```python
from build123d import *

# Parameters (mm, degrees)
F0_W        = 52.5702424347
F0_H        = 44.9169911444
F1_DEPTH    = 25
F2_DEPTH    = 25
F3_T        = -2.5
F4_SIZE     = 1
F5_T1_DEPTH = 68.9169911444
F5_T3_DEPTH = 6.1776694265
F5_T5_DEPTH = 48.0000001753
F5_T7_DEPTH = 6.1776694575
F5_T9_DEPTH = 75


# Not quite as in the source:
# - a fillet or chamfer that OpenCascade refuses, or shapes differently, is made with other operations: its cross-section is extruded or revolved along the edge and cut away or added


with BuildPart() as f1:
    # F0 (on Front) → F1 (new body)
    with BuildSketch(Plane.XZ):
        with Locations((26.2851212174, 22.4584955722)):
            Rectangle(F0_W, F0_H)
    extrude(amount=F1_DEPTH)

    # F2 (add): a face of the model
    f2_faces = [f1.faces().sort_by_distance(p)[0] for p in [
        (26.2851212174, -25, 22.4584955722),
    ]]
    extrude(f2_faces, amount=F2_DEPTH)

    # F3
    f3_openings = [f1.faces().sort_by_distance(p)[0] for p in [
        (26.285121, -25, 44.916991),
    ]]
    offset(amount=F3_T, openings=f3_openings)

    # F4
    f4_edges = [f1.edges().sort_by_distance(p)[0] for p in [
        (52.570242, 0, 22.458496),
        (52.570242, -25, 44.916991),
        (26.285121, -50, 44.916991),
        (0, -25, 44.916991),
        (26.285121, 0, 44.916991),
        (2.5, -25, 44.916991),
        (26.285121, -47.5, 44.916991),
        (50.070242, -25, 44.916991),
        (26.285121, -2.5, 44.916991),
    ]]
    chamfer(f4_edges, length=F4_SIZE)

    # F5: fillet of radius 5 on 4 edges, made by hand

    # F5_s2 → F5_t1 (cut)
    with BuildSketch(Plane.XY.offset(-12.5)):
        with BuildLine():
            ThreePointArc((0, -45), (1.4644660941, -48.5355339059), (5, -50))
            Line((5, -50), (0, -50))
            Line((0, -50), (0, -45))
        make_face()
        with BuildLine():
            ThreePointArc((0, -5), (1.4644660941, -1.4644660941), (5, 0))
            Line((5, 0), (0, 0))
            Line((0, 0), (0, -5))
        make_face()
    extrude(amount=F5_T1_DEPTH, mode=Mode.SUBTRACT)

    # F5_s4 → F5_t3 (cut)
    with BuildSketch(Plane.XZ.offset(49.0000001032)):
        with BuildLine():
            ThreePointArc((0, 41.8459233326), (0.3806023374, 43.7593404944), (1.4644660941, 45.3814572385))
            Line((1.4644660941, 45.3814572385), (0, 43.9169911444))
            Line((0, 43.9169911444), (0, 41.8459233326))
        make_face()
    extrude(amount=F5_T3_DEPTH, mode=Mode.SUBTRACT)

    # F5_s6 → F5_t5 (cut)
    with BuildSketch(Plane.XZ.offset(0.9999999279)):
        with BuildLine():
            ThreePointArc((0, 41.9169911444), (0.2565835097, 43.4981299745), (1, 44.9169911444))
            Line((1, 44.9169911444), (0, 43.9169911444))
            Line((0, 43.9169911444), (0, 41.9169911444))
        make_face()
    extrude(amount=F5_T5_DEPTH, mode=Mode.SUBTRACT)

    # F5_s8 → F5_t7 (cut)
    with BuildSketch(Plane.XZ.offset(-5.1776695297)):
        with BuildLine():
            ThreePointArc((0, 41.8459233326), (0.3806023374, 43.7593404944), (1.4644660941, 45.3814572385))
            Line((1.4644660941, 45.3814572385), (0, 43.9169911444))
            Line((0, 43.9169911444), (0, 41.8459233326))
        make_face()
    extrude(amount=F5_T7_DEPTH, mode=Mode.SUBTRACT)

    # F5_s10 → F5_t9 (cut)
    with BuildSketch(Plane.XZ.offset(-12.5)):
        with BuildLine():
            ThreePointArc((0, 5), (1.4644660941, 1.4644660941), (5, 0))
            Line((5, 0), (0, 0))
            Line((0, 0), (0, 5))
        make_face()
    extrude(amount=F5_T9_DEPTH, mode=Mode.SUBTRACT)


solid = f1.part
```
Read the model definition and answer for the solid it produces. Units are mm, in the model's axes. A direction names the side the tool comes from. Coordinates: 2 decimals unless noted, no trailing zeros. Write each loop counter-clockwise with the first axis right and the second up, starting at its lowest first coordinate (ties: lowest second). Pieces come first, ordered by that corner, then holes. Notation, with made-up numbers: (-32, 55) -> (-10, 55) arc R34 ccw to (-10, 85) -> close; hole circle Ø1 at (40, -0.5). An arc over 180 degrees is marked (long way). Answer as a JSON object with one key per item and string values.
Q1. The part is cut by section D-D on y = -4. Give the vertices of the cut face in (x, z).
The answers:
{"outline": "(0.1, 4) arc R5 ccw to (5, 0) -> (52.57, 0) -> (52.57, 43.92) -> (51.57, 44.92) -> (51.07, 44.92) -> (50.07, 43.92) -> (50.07, 2.5) -> (2.5, 2.5) -> (2.5, 43.92) -> (1.5, 44.92) -> (1, 44.92) arc R5 ccw to (0.1, 42.92) -> close"}
Q2. Consider line 1 (X direction, y = -42.5, z = 32); line 2 (Y direction, x = 16, z = 10.5); line 3 (Z direction, x = 6, y = -32). Determine where each line is inside the solid, lowest interval first. Write a range as [from, to].
The answers:
{"line 1": "x = [0, 2.5], [50.07, 52.57]", "line 2": "y = [-50, -47.5], [-2.5, 0]", "line 3": "z = [0, 2.5]"}
Q3. Flat-ended cylindrical pins translate along their axes: pin 1 Ø5 at (x, y) = (44, -8) entering from +Z; pin 2 Ø12 at (x, y) = (36.5, -26) entering from -Z. Find the tip coordinate at first contact, or state that the pin passes through.
The answers:
{"pin 1": "stops at z = 2.5", "pin 2": "stops at z = 0"}
Q4. Determine the mould class of faces 3 (the cylindrical face through (0.25, -24.68, 43.48)), 4 (the flat face through (28, -50, 22)), 5 (the flat face through (26, -25, 2.5)) for opening direction X: pulls with the +X half, pulls with the -X half, needs draft (parallel to the pull), parting line crosses it, or undercut.
The answers:
{"face 3": "pulls with the -X half", "face 4": "needs draft", "face 5": "undercut"}
Q5. A tool of negligible diameter and unlimited length cuts with its end or side. For faces 1 (the flat face through (26, -2.5, 23)), 2 (the flat face through (28, -25, 0)), from which of +Z, -Z, +X, -X, +Y, -Y can it reach the whole face along a straight path? Write none if from no direction.
The answers:
{"face 1": "+Z", "face 2": "-Z, +X, -X, +Y, -Y"}
Q6. The part is cut by section A-A on x = 8.5. Give the vertices of the cut face in (y, z).
The answers:
{"outline": "(-50, 0) -> (0, 0) -> (0, 43.92) -> (-1, 44.92) -> (-1.5, 44.92) -> (-2.5, 43.92) -> (-2.5, 2.5) -> (-47.5, 2.5) -> (-47.5, 43.92) -> (-48.5, 44.92) -> (-49, 44.92) -> (-50, 43.92) -> close"}
Q7. The part is cut by section C-C on y = -37. Give the vertices of the cut face in (x, z), then the cut area to 3 significant figures.
The answers:
{"outline": "(0, 5) arc R5 ccw to (5, 0) -> (52.57, 0) -> (52.57, 43.92) -> (51.57, 44.92) -> (51.07, 44.92) -> (50.07, 43.92) -> (50.07, 2.5) -> (2.5, 2.5) -> (2.5, 43.92) -> (1.5, 44.92) -> (1, 44.92) arc R5 ccw to (0, 41.92) -> close", "area": "336 mm2"}
Q8. The part is cut by section B-B on z = 37. Give the vertices of the cut face in (x, y), then the cut area to 3 significant figures.
The answers:
{"outline": "(0, -45) arc R5 ccw to (5, -50) -> (52.57, -50) -> (52.57, -1) -> (51.57, 0) -> (5, 0) arc R5 ccw to (0, -5) -> close; hole (2.5, -47.5) -> (50.07, -47.5) -> (50.07, -2.5) -> (2.5, -2.5) -> close", "area": "477 mm2"}
